Can you work these out from the model? Positions are in its coordinate system, mm. A direction names the side the tool comes from. Give positions to 0.01 mm unless a question says otherwise; leave off trailing zeros. Order: outer loops, then holes, each group sorted by start corner. A loop starts at its lowest first (then second) coordinate and runs counter-clockwise, first axis right, second up. Notation, with made-up numbers: M 40.5,-5.75 L 53.5,-5.75 A12 ccw 53.5,8.25 Z; hole C -7.75,38.25 d7. An arc over 180 degrees is marked long. Write each question's results on one line, items separated by ' | '.
Autodesk Fusion 360 part; units mm, degrees
sketch "Sketch1" plane through (0, 0, 0) normal (0, 0, 1) x (1, 0, 0)
  line L0 (-1.25, 17.5) -> (1.25, 17.5)
  line L1 (1.25, 17.5) -> (1.25, -17.5)
  line L2 (1.25, -17.5) -> (-1.25, -17.5)
  line L3 (-1.25, -17.5) -> (-1.25, 17.5)
  line L4 (-1.25, 17.5) -> (1.25, -17.5) construction
  line L5 (1.25, 17.5) -> (-1.25, -17.5) construction
  line L6 (0, 0) -> (0, -14.0845) construction
  line L7 (-1.25, -14.8345) -> (-13.75, -14.8345)
  line L8 (-13.75, -14.8345) -> (-13.75, -13.3345)
  line L9 (-13.75, -13.3345) -> (-1.25, -13.3345)
  line L10 (1.25, -0.775) -> (6.25, -0.775)
  line L11 (6.25, -0.775) -> (6.25, 0.725)
  line L12 (6.25, 0.725) -> (1.25, 0.725)
  line L13 (0, -14.0845) -> (-12.5, -14.0845) construction
  line L14 (0, 0) -> (-10.5, 0) construction
  line L15 (-13.75, 13.3345) -> (-1.25, 13.3345)
  line L16 (-1.25, 14.8345) -> (-13.75, 14.8345)
  line L17 (-13.75, 13.3345) -> (-13.75, 14.8345)
  line L18 (-1.25, 17.5) -> (-1.25, 25)
  line L19 (1.25, 17.5) -> (1.25, 25)
  line L20 (1.25, 25) -> (-1.25, 25)
  dimension "d1" = 35
  dimension "d2" = 14.0845
  dimension "d3" = 0.75
  dimension "d4" = 1.5
  dimension "d5" = 12.5
  dimension "d6" = 1.5
  dimension "d7" = 0.775
  dimension "d8" = 5
  dimension "d9" = 2.5
  dimension "d10" = 12.5
  dimension "d19" = 7.5
  dimension "d20" = 7.5
extrude "Extrude1" add sketch "Sketch1" along normal blind 1.5
fillet "Fillet1" radius 0.25 4 edges at (3.75, -0.775, 1.5) (3.75, -0.775, 0) (3.75, 0.725, 0) (3.75, 0.725, 1.5)
fillet "Fillet2" radius 0.25 4 edges at (-7.5, -14.8345, 1.5) (-7.5, -13.3345, 1.5) (-7.5, -13.3345, 0) (-7.5, -14.8345, 0)
fillet "Fillet3" radius 0.25 4 edges at (-7.5, 14.8345, 1.5) (-7.5, 13.3345, 1.5) (-7.5, 14.8345, 0) (-7.5, 13.3345, 0)
fillet "Fillet4" radius 0.25 16 edges at (-13.75, -14.8345, 0.75) (-13.75, -14.7613, 0.0732) (-13.75, -14.0845, 0) (-13.75, -13.4077, 0.0732) (-13.75, -13.3345, 0.75) (-13.75, -13.4077, 1.4268) (-13.75, -14.0845, 1.5) (-13.75, -14.7613, 1.4268) (-13.75, 13.3345, 0.75) (-13.75, 13.4077, 0.0732) (-13.75, 14.0845, 0) (-13.75, 14.7613, 0.0732) (-13.75, 14.8345, 0.75) (-13.75, 14.7613, 1.4268) (-13.75, 14.0845, 1.5) (-13.75, 13.4077, 1.4268)
equation "d2 = ( 28.169 / 2 ) * 1 mm"
equation "d3 = ( 1.5 / 2 ) * 1 mm"
equation "d7 = ( 1.55 / 2 ) * 1 mm"
(1) Imagine slicing it at A-A, the plane x = -3.75. Write out the boundary of the cut face in (y, z), plus the area to 3 significant figures.
Data:
outline: M -14.83,0.25 A0.25 ccw -14.58,0 L -13.58,0 A0.25 ccw -13.33,0.25 L -13.33,1.25 A0.25 ccw -13.58,1.5 L -14.58,1.5 A0.25 ccw -14.83,1.25 Z; M 13.33,0.25 A0.25 ccw 13.58,0 L 14.58,0 A0.25 ccw 14.83,0.25 L 14.83,1.25 A0.25 ccw 14.58,1.5 L 13.58,1.5 A0.25 ccw 13.33,1.25 Z | area: 4.39 mm2
(2) I need wall thicknesses on L1, parallel to Y at x = -7.5, z = 1.25; L2, parallel to X at y = -9, z = 0.75; L3, parallel to Y at x = -9.5, z = 1.4. Which ranges of each line are inside material? Lowest first, please. Write a range as from..to.
Data:
L1: y = -14.83..-13.33, 13.33..14.83 | L2: x = -1.25..1.25 | L3: y = -14.78..-13.38, 13.38..14.78
(3) Will these pins go through, and if not, where does the flat tip stop? P1, Ø0.8, axis at y = -16.5, z = 1, coming from the -X side; P2, Ø1.5, axis at x = -11.5, y = 12.5, coming from the -Z side; P3, Ø0.5, axis at x = 4.5, z = 1, coming from the -Y side (3 decimals); P4, Ø3, axis at x = -9.5, y = -12.5, coming from the -Z side.
Data:
P1: stops at x = -1.25 | P2: passes through | P3: stops at y = -0.775 | P4: stops at z = 0
(4) Imagine slicing it at C-C, the plane x = 4.5. Write out the boundary of the cut face in (y, z) (3 decimals).
Data:
outline: M -0.775,0.25 A0.25 ccw -0.525,0 L 0.475,0 A0.25 ccw 0.725,0.25 L 0.725,1.25 A0.25 ccw 0.475,1.5 L -0.525,1.5 A0.25 ccw -0.775,1.25 Z
(5) Imagine slicing it at D-D, the plane y = -6.5. Write out the boundary of the cut face in (x, z), plus the area to 3 significant figures.
Data:
outline: M -1.25,0 L 1.25,0 L 1.25,1.5 L -1.25,1.5 Z | area: 3.75 mm2
(6) For faces 1 (the face through (1.25, 13, 1)), 2 (the face through (-7, 14.834, 1)), 3 (the face through (-7, -14.834, 1)), 4 (the face through (4, -0.775, 1)), 5 (the face through (-7, -13.334, 1)), which set-ups out of +Z, -Z, +X, -X, +Y, -Y let a thin tool reach every point of the face, with its end or its side?
Data:
face 1: +Z, -Z, +X, +Y | face 2: +Z, -Z, -X, +Y | face 3: +Z, -Z, -X, -Y | face 4: +Z, -Z, +X, -Y | face 5: +Z, -Z, -X
